Geometry check sheet. Reference: drawing and pictorial views, mm from the part's lowest x, y, z. A direction names the side the tool comes from. Round coordinates to 2 decimals unless told otherwise and drop trailing zeros. Write each loop counter-clockwise with the first axis right and the second up, starting at its lowest first coordinate (ties: lowest second). Pieces come first, ordered by that corner, then holes. Notation, with made-up numbers: M 78,-3.75 L 97,-3.75 A17 cw 97,3.25 Z; hole C 83.25,68.5 d3. An arc over 180 degrees is marked long. Answer in a Markdown table with one row per item. Add a question column.
1. Sectioned sample at A-A on x = 53. Record the cut outline in (y, z) (1 decimal).
2. Sectioned sample at D-D on x = 40. Record the cut outline in (y, z) (1 decimal), plus the area to 3 significant figures.
3. Set-up check for the marked faces 5, 6, 7 and 8: record each of +Z, -Z, +X, -X, +Y, -Y from which the full face is reachable in a straight line by a thin tool's end or side.
4. Draft check along X on the marked faces 1, 2, 3 and 4. Enter one of: pulls with the +X half, pulls with the -X half, needs draft (parallel to the pull), parting line crosses it, or undercut.
5. Material ranges on probe 1 along X at (y, z) = (50, 25); probe 2 along X at (y, z) = (49.5, 67.5); probe 3 along X at (y, z) = (84.5, 5), recorded low to high.
6. Sectioned sample at B-B on z = 27.5. Record the cut outline in (x, y) (1 decimal).
7. Go/stop test with flat-tipped pins: pin 1 Ø10 at (y, z) = (16, 39.5) entering from +X; pin 2 Ø20.5 at (x, y) = (54.5, 50.8) entering from +Z; pin 3 Ø10 at (y, z) = (8.5, 50) entering from -X; pin 4 Ø6.5 at (x, y) = (51, 5.5) entering from +Z (3 decimals). Record where each tip stops, or that it passes through.
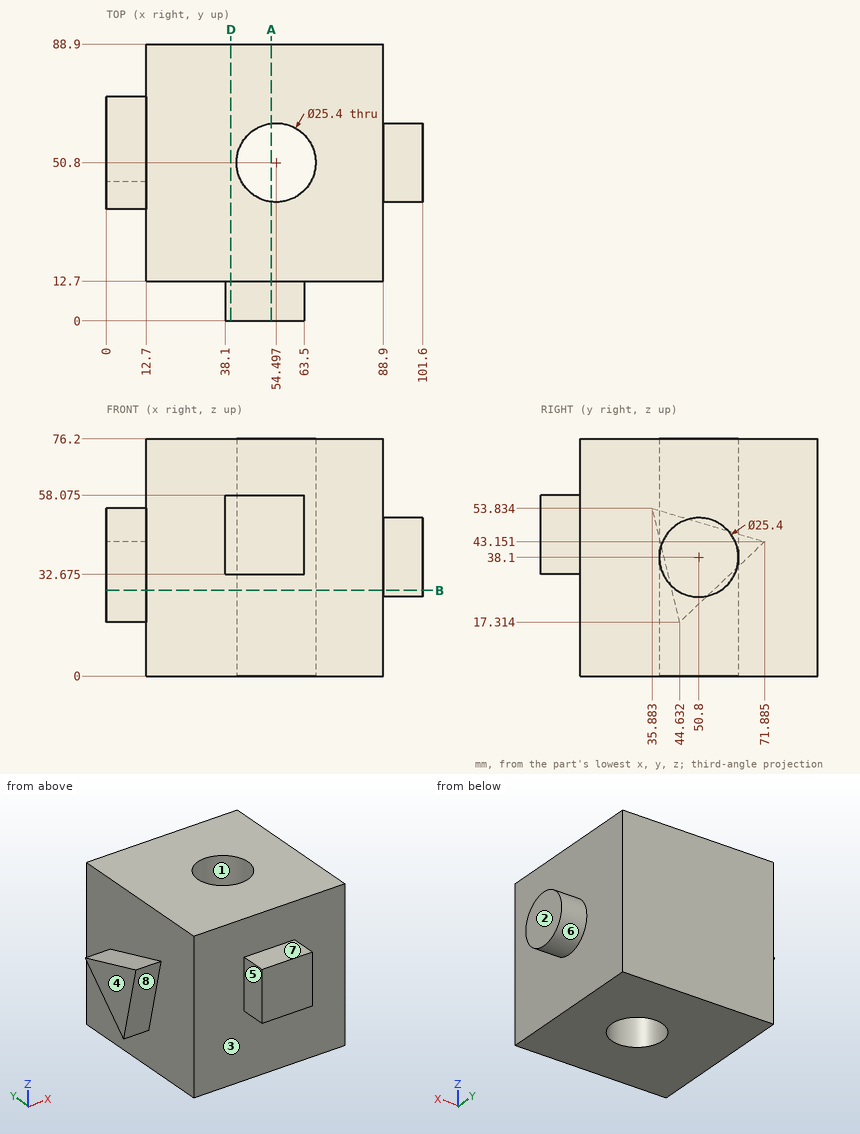
Geometry check:
| question | item | result |
|---|---|---|
| 1 | outline | M 0,32.7 L 12.7,32.7 L 12.7,0 L 38.2,0 L 38.2,76.2 L 12.7,76.2 L 12.7,58.1 L 0,58.1 Z; M 63.4,0 L 88.9,0 L 88.9,76.2 L 63.4,76.2 Z |
| 2 | outline | M 0,32.7 L 12.7,32.7 L 12.7,0 L 88.9,0 L 88.9,76.2 L 12.7,76.2 L 12.7,58.1 L 0,58.1 Z |
| 2 | area | 6,130 mm2 |
| 3 | face 5 | +Z, -Z, -X, -Y |
| 3 | face 6 | +X |
| 3 | face 7 | +Z, +X, -X, -Y |
| 3 | face 8 | -Z, -X, -Y |
| 4 | face 1 | undercut |
| 4 | face 2 | pulls with the +X half |
| 4 | face 3 | needs draft |
| 4 | face 4 | pulls with the -X half |
| 5 | probe 1 | x = 0 to 41.82, 67.17 to 88.9 |
| 5 | probe 2 | x = 12.7 to 41.86, 67.13 to 88.9 |
| 5 | probe 3 | x = 12.7 to 88.9 |
| 6 | outline | M 0,42.2 L 12.7,42.2 L 12.7,12.7 L 88.9,12.7 L 88.9,43.8 L 101.6,43.8 L 101.6,57.8 L 88.9,57.8 L 88.9,88.9 L 12.7,88.9 L 12.7,55.4 L 0,55.4 Z; hole C 54.5,50.8 d25.4 |
| 7 | pin 1 | stops at x = 88.9 |
| 7 | pin 2 | passes through |
| 7 | pin 3 | stops at x = 12.7 |
| 7 | pin 4 | stops at z = 58.075 |
